Design review of the part built by this model. Coordinates are the model's own, in mm. A direction names the side the tool comes from. Give positions to 0.01 mm unless a question says otherwise; leave off trailing zeros. Order: outer loops, then holes, each group sorted by start corner. A loop starts at its lowest first (then second) coordinate and runs counter-clockwise, first axis right, second up. Notation, with made-up numbers: (57.25, 15.25) - (91.25, 15.25) arc R16 ccw to (91.25, 22.25) - close; hole circle Ø2 at (56, -6). An arc over 180 degrees is marked (long way). Write each question's results on one line, items separated by ' | '. Start each with the question number.
```python
from build123d import *

# Parameters (mm, degrees)
SKETCH1_W                    = 35
SKETCH1_H                    = 35
BASE_FLANGE1_DEPTH           = 1.5
EDGE_FLANGE1_STRIP_W         = 7.4732
EDGE_FLANGE1_STRIP_H         = 1.5
EDGE_FLANGE1_STRIP_CUT_DEPTH = 35
EDGE_FLANGE1_DEPTH           = 35
CUT_EXTRUDE1_REACH           = 62.39
SKETCH9_R                    = 1.5
CUT_EXTRUDE2_REACH           = 122.529
SKETCH10_R                   = 1


# Sheet-metal steps are written as plain solids
with BuildPart() as part:
    # Sketch1 → Base-Flange1 (new body)
    with BuildSketch(Plane(origin=(0, 12.100921456, 0), x_dir=(1, 0, 0), z_dir=(0, 1, 0))):
        with Locations((-96.5, 0)):
            Rectangle(SKETCH1_W, SKETCH1_H)
    extrude(amount=BASE_FLANGE1_DEPTH)

    # Edge-Flange1 strip (across the edge) → Edge-Flange1 strip cut (cut)
    with BuildSketch(Plane(origin=(-79, 13.600921456, 17.5), x_dir=(-1, 0, 0), z_dir=(0, 0, -1))):
        with Locations((-1.5, -0.75)):
            Rectangle(EDGE_FLANGE1_STRIP_W, EDGE_FLANGE1_STRIP_H)
    extrude(amount=EDGE_FLANGE1_STRIP_CUT_DEPTH, mode=Mode.SUBTRACT)

    # Edge-Flange1 section (across the edge) → Edge-Flange1 (add)
    with BuildSketch(Plane(origin=(-79, 13.600921456, 17.5), x_dir=(-1, 0, 0), z_dir=(0, 0, -1))):
        with BuildLine():
            Line((0, 0.7366), (0, 33.5))
            Line((0, 33.5), (1.5, 33.5))
            Line((1.5, 33.5), (1.5, 0.7366))
            ThreePointArc((1.5, 0.7366), (1.715745145, 0.215745145), (2.2366, 0))
            Line((2.2366, 0), (2.2366, -1.5))
            ThreePointArc((2.2366, -1.5), (0.655084973, -0.844915027), (0, 0.7366))
        make_face()
    extrude(amount=EDGE_FLANGE1_DEPTH)

    # Sketch9 → Cut-Extrude1 (cut, up to next)
    with BuildSketch(Plane.ZY.offset(80.5), mode=Mode.PRIVATE) as cut_extrude1_sk1:
        with Locations(Location((-11.5, 39.145, 0), (0, 0, 270))):
            Circle(SKETCH9_R)
    cut_extrude1_tool1 = extrude(cut_extrude1_sk1.sketch, amount=-CUT_EXTRUDE1_REACH, mode=Mode.PRIVATE) & part.part
    # Sketch9 → Cut-Extrude1 (cut, up to next)
    with BuildSketch(Plane.ZY.offset(80.5), mode=Mode.PRIVATE) as cut_extrude1_sk2:
        with Locations(Location((11.5, 39.145, 0), (0, 0, 270))):
            Circle(SKETCH9_R)
    cut_extrude1_tool2 = extrude(cut_extrude1_sk2.sketch, amount=-CUT_EXTRUDE1_REACH, mode=Mode.PRIVATE) & part.part
    # Sketch9 → Cut-Extrude1 (cut, up to next)
    with BuildSketch(Plane.ZY.offset(80.5), mode=Mode.PRIVATE) as cut_extrude1_sk3:
        with Locations(Location((11.5, 18.578902177, 0), (0, 0, 270))):
            Circle(SKETCH9_R)
    cut_extrude1_tool3 = extrude(cut_extrude1_sk3.sketch, amount=-CUT_EXTRUDE1_REACH, mode=Mode.PRIVATE) & part.part
    # Sketch9 → Cut-Extrude1 (cut, up to next)
    with BuildSketch(Plane.ZY.offset(80.5), mode=Mode.PRIVATE) as cut_extrude1_sk4:
        with Locations(Location((-11.5, 18.578902177, 0), (0, 0, 270))):
            Circle(SKETCH9_R)
    cut_extrude1_tool4 = extrude(cut_extrude1_sk4.sketch, amount=-CUT_EXTRUDE1_REACH, mode=Mode.PRIVATE) & part.part
    add(cut_extrude1_tool1.solids().sort_by_distance((-80.5, 39.145, -11.5))[0], mode=Mode.SUBTRACT)
    add(cut_extrude1_tool2.solids().sort_by_distance((-80.5, 39.145, 11.5))[0], mode=Mode.SUBTRACT)
    add(cut_extrude1_tool3.solids().sort_by_distance((-80.5, 18.578902, 11.5))[0], mode=Mode.SUBTRACT)
    add(cut_extrude1_tool4.solids().sort_by_distance((-80.5, 18.578902, -11.5))[0], mode=Mode.SUBTRACT)

    # Sketch10 → Cut-Extrude2 (cut, up to next)
    with BuildSketch(Plane.XZ.offset(-12.100921456), mode=Mode.PRIVATE) as cut_extrude2_sk1:
        with Locations(Location((-97.512607475, -7.747, 0), (0, 0, 270))):
            Circle(SKETCH10_R)
    cut_extrude2_tool1 = extrude(cut_extrude2_sk1.sketch, amount=-CUT_EXTRUDE2_REACH, mode=Mode.PRIVATE) & part.part
    # Sketch10 → Cut-Extrude2 (cut, up to next)
    with BuildSketch(Plane.XZ.offset(-12.100921456), mode=Mode.PRIVATE) as cut_extrude2_sk2:
        with Locations(Location((-97.512607475, 7.747, 0), (0, 0, 270))):
            Circle(SKETCH10_R)
    cut_extrude2_tool2 = extrude(cut_extrude2_sk2.sketch, amount=-CUT_EXTRUDE2_REACH, mode=Mode.PRIVATE) & part.part
    add(cut_extrude2_tool1.solids().sort_by_distance((-97.512607, 12.100921, -7.747))[0], mode=Mode.SUBTRACT)
    add(cut_extrude2_tool2.solids().sort_by_distance((-97.512607, 12.100921, 7.747))[0], mode=Mode.SUBTRACT)


solid = part.part
```
Q1. Machinability: for faces 4 (the flat face through (-98, 13.601, 0)), 5 (the flat face through (-80, 22, 17.5)), which of the approach directions +Z, -Z, +X, -X, +Y, -Y give a long, thin tool a straight path to every point of the face, cutting with its end or side? Answer none if there is none.
Q2. Add section A-A (z = -11.5). Give the boundary of the cut face in (x, y) (3 decimals), plus the area to 3 significant figures.
Q3. For line 1 (X direction, y = 36, z = -9); line 2 (Y direction, x = -93, z = -0.5), list the stretches that pass through material, from the lowest coordinate up. Write a range as [from, to].
Q4. Draft analysis for pull direction X (two halves, no side actions). For faces 1 (the flat face through (-79, 30, 0)), 2 (the flat face through (-80.5, 31, 0)), 3 (the cylindrical face through (-98.4, 12.84, 7.29)), state which applies: pulls with the +X half, pulls with the -X half, needs draft (parallel to the pull), parting line crosses it, or undercut.
Q5. Insertion check: pin 1 Ø4 at (y, z) = (18.58, 11.5) entering from -X; pin 2 Ø16.5 at (x, z) = (-92.5, 6) entering from +Y. Each pin has a flat end and moves straight along its axis. Give the tip position at first contact, or say it passes through.
Q6. Add section B-B (z = -6). Give the boundary of the cut face in (x, y).
Q7. Add section C-C (z = 8). Give the boundary of the cut face in (x, y).
Q8. Add section D-D (y = 27.5). Give the boundary of the cut face in (x, z), plus the area to 3 significant figures.
Verdict:
1) face 4: +Z, -Z, -X, +Y | face 5: +Z, +X, -X, +Y, -Y
2) outline: (-114, 12.101) - (-81.237, 12.101) arc R2.237 ccw to (-79, 14.338) - (-79, 17.079) - (-80.5, 17.079) - (-80.5, 14.338) arc R0.737 cw to (-81.237, 13.601) - (-114, 13.601) - close; (-80.5, 20.079) - (-79, 20.079) - (-79, 37.645) - (-80.5, 37.645) - close; (-80.5, 40.645) - (-79, 40.645) - (-79, 47.101) - (-80.5, 47.101) - close | area: 92.8 mm2
3) line 1: x = [-80.5, -79] | line 2: y = [12.1, 13.6]
4) face 1: pulls with the +X half | face 2: pulls with the -X half | face 3: undercut
5) pin 1: stops at x = -80.5 | pin 2: stops at y = 13.6
6) outline: (-114, 12.1) - (-81.24, 12.1) arc R2.24 ccw to (-79, 14.34) - (-79, 47.1) - (-80.5, 47.1) - (-80.5, 14.34) arc R0.74 cw to (-81.24, 13.6) - (-114, 13.6) - close
7) outline: (-114, 12.1) - (-98.48, 12.1) - (-98.48, 13.6) - (-114, 13.6) - close; (-96.55, 12.1) - (-81.24, 12.1) arc R2.24 ccw to (-79, 14.34) - (-79, 47.1) - (-80.5, 47.1) - (-80.5, 14.34) arc R0.74 cw to (-81.24, 13.6) - (-96.55, 13.6) - close
8) outline: (-80.5, -17.5) - (-79, -17.5) - (-79, 17.5) - (-80.5, 17.5) - close | area: 52.5 mm2
